```python
from build123d import *

# Parameters (mm, degrees)
SKETCH_1_R          = 4
EXTRUDE_1_DEPTH     = 39.5
SKETCH_2_R          = 3
EXTRUDE_2_DEPTH     = 1
SKETCH_3_R          = 4
EXTRUDE_3_DEPTH     = 707.5
SKETCH_4_R          = 3
EXTRUDE_4_DEPTH     = 42.5
CHAMFER_1_SIZE      = 1.5
CUT_EXTRUDE_1_DEPTH = 5


with BuildPart() as part:
    # 草图1 → 凸台-拉伸1 (new body)
    with BuildSketch(Plane(origin=(0, 0, 0), x_dir=(0, 0, -1), z_dir=(1, 0, 0))):
        Circle(SKETCH_1_R)
    extrude(amount=EXTRUDE_1_DEPTH)

    # 草图2 → 凸台-拉伸2 (add)
    with BuildSketch(Plane(origin=(39.5, 0, 0), x_dir=(0, 0, -1), z_dir=(1, 0, 0))):
        Circle(SKETCH_2_R)
    extrude(amount=EXTRUDE_2_DEPTH)

    # 草图3 → 凸台-拉伸3 (add)
    with BuildSketch(Plane(origin=(40.5, 0, 0), x_dir=(0, 0, -1), z_dir=(1, 0, 0))):
        Circle(SKETCH_3_R)
    extrude(amount=EXTRUDE_3_DEPTH)

    # 草图4 → 凸台-拉伸4 (add)
    with BuildSketch(Plane(origin=(748, 0, 0), x_dir=(0, 0, -1), z_dir=(1, 0, 0))):
        Circle(SKETCH_4_R)
    extrude(amount=EXTRUDE_4_DEPTH)

    # 倒角1
    chamfer_1_edges = [part.edges().sort_by_distance(p)[0] for p in [
        (790.5, 0, 3),
    ]]
    chamfer(chamfer_1_edges, length=CHAMFER_1_SIZE)

    # 草图7 → 切除-拉伸1 (cut)
    with BuildSketch(Plane.ZY):
        Polygon((-2.38156986, 1.375), (-2.38156986, -1.375), (0, -2.75), (2.38156986, -1.375), (2.38156986, 1.375), (0, 2.75), align=None)
    extrude(amount=-CUT_EXTRUDE_1_DEPTH, mode=Mode.SUBTRACT)


solid = part.part
```
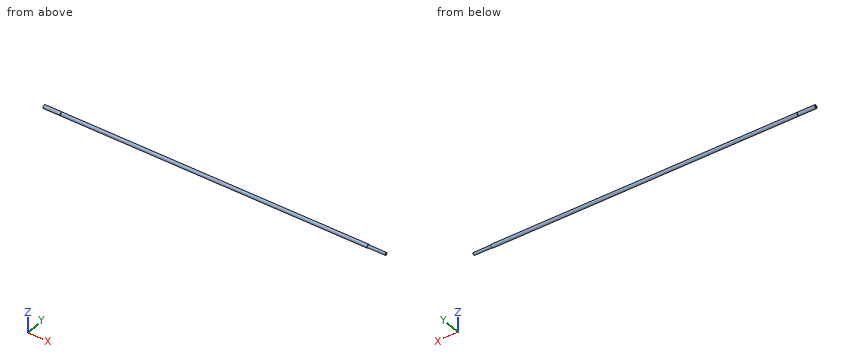
Model file for the job. Use its own axes, mm. Coordinates: 2 decimals unless noted, no trailing zeros. Order: outer loops, then holes, each group sorted by start corner. A loop starts at its lowest first (then second) coordinate and runs counter-clockwise, first axis right, second up. Notation, with made-up numbers: M -36,-27.5 L 13,-27.5 A21 cw 13,2.5 Z; hole C 30.5,1 d6. An arc over 180 degrees is marked long. Answer as CSV lines item,"result".
(1) Flat gauge pin, fed straight in: pin 1 (1.5 mm diameter, centred on x = 95.5, y = -1, fed in from -Z). Where does the tip first touch, or does it go through?
Geometry says:
pin 1,"stops at z = -3.99"
(2) Wall check: line 1 along X through (y, z) = (-3.25, -2); line 2 along Y through (x, z) = (66, 3.25); line 3 along X through (y, z) = (0.5, 0.25). Give the ranges that are in metal, low to high.
Geometry says:
line 1,"x = 0 to 39.5, 40.5 to 748"
line 2,"y = -2.33 to 2.33"
line 3,"x = 5 to 790.5"
(3) Band-saw the part on A-A, the plane y = 0. List the corners of the cut face in (x, z), then the cut area to 3 significant figures.
Geometry says:
outline,"M 0,-4 L 39.5,-4 L 39.5,-3 L 40.5,-3 L 40.5,-4 L 748,-4 L 748,-3 L 789,-3 L 790.5,-1.5 L 790.5,1.5 L 789,3 L 748,3 L 748,4 L 40.5,4 L 40.5,3 L 39.5,3 L 39.5,4 L 0,4 L 0,2.38 L 5,2.38 L 5,-2.38 L 0,-2.38 Z"
area,"6,210 mm2"
(4) Band-saw the part on B-B, the plane x = 420. List the corners of the cut face in (y, z), then the cut area to 3 significant figures.
Geometry says:
outline,"C 0,0 d8"
area,"50.3 mm2"
